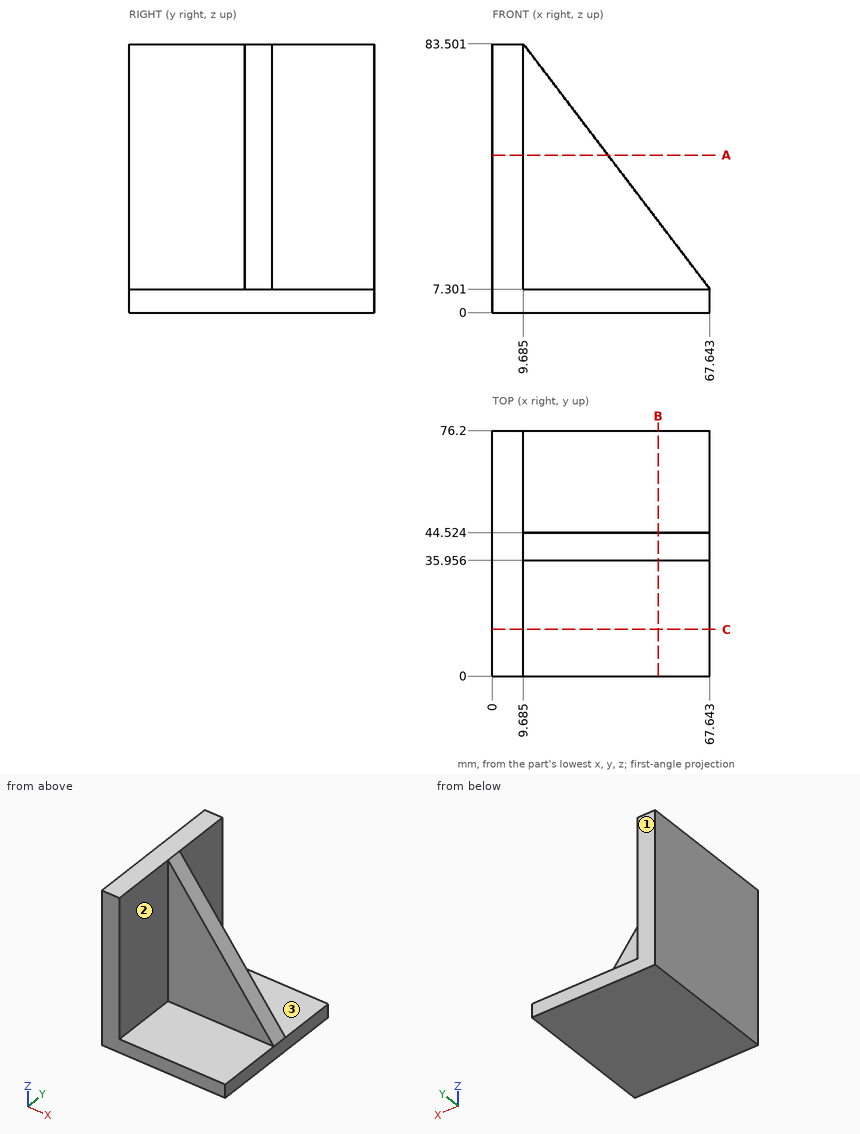
Input: dimensioned drawing with shaded views. Units: mm. Origin: part minimum x, y, z. A direction names the side the tool comes from. Give positions to 0.01 mm unless a question says otherwise; leave off trailing zeros. Order: outer loops, then holes, each group sorted by start corner. A loop starts at its lowest first (then second) coordinate and runs counter-clockwise, first axis right, second up. Notation, with made-up numbers: (54, 20) -> (64, 20) arc R25 ccw to (64, 55) -> close; hole circle Ø6 at (42.25, -14.75). An arc over 180 degrees is marked (long way). Answer as a JSON object with one key per item and string values.
Q1. Access query for the marked faces 1, 2 and 3. Directions: +Z, -Z, +X, -X, +Y, -Y. A direction counts if a zero-diameter tool reaches every point of the face in a straight line with its end or side. Return the directions, or none.
Entries:
{"face 1": "+Z, -Z, +X, -X, +Y", "face 2": "+Z, +X, -Y", "face 3": "+Z, +X, +Y"}
Q2. Section C-C (y = 14.5). Output: boundary loops of the cut face in (x, z) (1 decimal), plus the area to 3 significant figures.
Entries:
{"outline": "(0, 0) -> (67.6, 0) -> (67.6, 7.3) -> (9.7, 7.3) -> (9.7, 83.5) -> (0, 83.5) -> close", "area": "1,230 mm^2"}
Q3. Section B-B (x = 51.5). Output: boundary loops of the cut face in (y, z) (1 decimal), plus the area to 3 significant figures.
Entries:
{"outline": "(0, 0) -> (76.2, 0) -> (76.2, 7.3) -> (44.5, 7.3) -> (44.5, 28.5) -> (36, 28.5) -> (36, 7.3) -> (0, 7.3) -> close", "area": "738 mm^2"}
Q4. First-contact query: pin 1 (17.5 mm diameter, centred on x = 42.5, z = 43, fed in from -Y); pin 2 (4 mm diameter, centred on y = 63.5, z = 40, fed in from +X) (1 decimal); pin 3 (11 mm diameter, centred on x = 25, y = 20.5, fed in from +Z). Flat tips, straight axial feed; report the tip coordinate or a pass-through.
Entries:
{"pin 1": "stops at y = 35.96", "pin 2": "stops at x = 9.7", "pin 3": "stops at z = 7.3"}
Q5. Section A-A (z = 49). Output: boundary loops of the cut face in (x, y) (1 decimal).
Entries:
{"outline": "(0, 0) -> (9.7, 0) -> (9.7, 36) -> (35.9, 36) -> (35.9, 44.5) -> (9.7, 44.5) -> (9.7, 76.2) -> (0, 76.2) -> close"}
Q6. Material intervals for probe 1 along X at (y, z) = (35.5, 24) (1 decimal); probe 2 along Y at (x, z) = (26.5, 16) (1 decimal); probe 3 along Z at (x, y) = (48, 59.5), sorted ascending.
Entries:
{"probe 1": "x = 0 to 9.7", "probe 2": "y = 36 to 44.5", "probe 3": "z = 0 to 7.3"}
